Read the model definition and answer for the solid it produces. Units are mm, in the model's axes. Face numbers are marked on the shaded views. A direction names the side the tool comes from. Coordinates: 2 decimals unless noted, no trailing zeros. Write each loop counter-clockwise with the first axis right and the second up, starting at its lowest first coordinate (ties: lowest second). Pieces come first, ordered by that corner, then holes.
(1) Which of the six approach directions +Z, -Z, +X, -X, +Y, -Y give full straight-line access (tool end or side, diameter ignored) to the marked faces 5, 6, 7 and 8?
(2) Section A-A on y = 7.75 is taken. Write down the section's boundary in (x, z).
(3) Given pin 1 (0.5 mm diameter, centred on x = 5.5, y = 1, fed in from -Z); pin 2 (3 mm diameter, centred on y = 10, z = -1, fed in from +X); pin 3 (2 mm diameter, centred on x = 2, y = 8, fed in from -Z); pin 4 (6 mm diameter, centred on y = 1.5, z = 2, fed in from -X), each flat-ended and moving along its own axis, determine where each tip first touches the part or whether it passes through.
(4) Section B-B on z = 2.25 is taken. Write down the section's boundary in (x, y).
(5) The mould has two halves that part along X. Classify the marked faces 1, 2, 3 and 4: +X half, -X half, draft (parallel to the pull), parting line (faces both ways), or undercut.
(6) Section D-D on y = 5.25 is taken. Write down the section's boundary in (x, z), then the cut area to 3 significant figures.
(7) Section C-C on x = 7.25 is taken. Write down the section's boundary in (y, z).
(8) Find the intervals of material crossed by probe 1 along Y at (x, z) = (-2.55, -0.25); probe 2 along X at (y, z) = (3.25, -1.25); probe 3 along Z at (x, y) = (-1.5, 7.5), in increasing order.
Autodesk Inventor part; units mm, degrees
ref_plane "YZ Plane" through (0, 0, 0) normal (1, 0, 0) x (0, 1, 0)
ref_plane "XZ Plane" through (0, 0, 0) normal (0, 1, 0) x (-1, 0, 0)
ref_plane "XY Plane" through (0, 0, 0) normal (0, 0, 1) x (1, 0, 0)
sketch "Sketch1" plane through (0, 0, 0) normal (0, 1, 0) x (-1, 0, 0)
  circle A0 centre (6, 0) radius 1.6
  circle A1 centre (6, 0) radius 1.6
  circle A2 centre (-6, 0) radius 1.6
  circle A3 centre (-6, 0) radius 1.6
  line L0 (1, 2.75) -> (1, -2.75) construction
  line L1 (1, 2.75) -> (-1, 2.75)
  line L2 (-1, -2.75) -> (-1, 2.75) construction
  line L3 (-1, -2.75) -> (1, -2.75)
  line L4 (0, 2.75) -> (0, -2.75) construction
  line L5 (-1, -2.75) -> (-3, -2.75)
  line L6 (-3, -2.75) -> (-3, 2.75)
  line L7 (-3, 2.75) -> (-1, 2.75)
  line L8 (-1, 2.75) -> (-1, -2.75)
  line L9 (1, -2.75) -> (3, -2.75)
  line L10 (3, -2.75) -> (3, 2.75)
  line L11 (3, 2.75) -> (1, 2.75)
  line L12 (1, 2.75) -> (1, -2.75)
  line L13 (6, 0) -> (-6, 0) construction
  arc A4 (6, -2.5) -> (6, 2.5) centre (6, 0) ccw
  arc A5 (-6, 2.5) -> (-6, -2.5) centre (-6, 0) ccw
  line L14 (0, 2.75) -> (0, -2.75) construction
  arc A6 (4, 2.75) -> (-4, 2.75) centre (0, 2.75) ccw
  arc A7 (-4, -2.75) -> (4, -2.75) centre (0, -2.75) ccw
  line L15 (4, -2.75) -> (4, -2.5)
  line L16 (4, 2.5) -> (4, 2.75)
  line L17 (-4, 2.75) -> (-4, 2.5)
  line L18 (-4, -2.5) -> (-4, -2.75)
  line L19 (-6, -2.5) -> (-4, -2.5)
  line L20 (4, -2.5) -> (6, -2.5)
  line L21 (6, 2.5) -> (4, 2.5)
  line L22 (-4, 2.5) -> (-6, 2.5)
  point P0 (0, 0)
  point P1 (0, 0)
  point P2 (0, 0)
  point P3 (0, 0)
  point P4 (0, 0)
  point P5 (0, 0)
  dimension "d6" = 2
  dimension "d7" = 2
  dimension "d8" = 5
  dimension "d9" = 8
extrude "Extrusion1" add sketch "Sketch1" along normal blind 2 contours L11 L10 L9 L12 | L8 L5 L6 L7 | L20 L15 A7 L18 L19 A5 L22 L17 A6 L16 L21 A4
fillet "Fillet1" radius 1 4 edges at (4, 1, -2.5) (4, 1, 2.5) (-4, 1, -2.5) (-4, 1, 2.5)
sketch "Sketch3" plane through (0, 2, 0) normal (0, 1, 0) x (1, 0, 0)
  line L0 (1, -2.75) -> (-1, -2.75)
  line L1 (1, -2.75) -> (3, -2.75)
  line L2 (3, -2.75) -> (3, 2.75)
  line L3 (3, 2.75) -> (1, 2.75)
  line L4 (1, 2.75) -> (1, -2.75)
  line L5 (-1, -2.75) -> (-3, -2.75)
  line L6 (-3, -2.75) -> (-3, 2.75)
  line L7 (-3, 2.75) -> (-1, 2.75)
  line L8 (-1, 2.75) -> (-1, -2.75)
  point P0 (0, 0)
  dimension "d11" = 2
  dimension "d12" = 5.5
  dimension "d13" = 2
extrude "Extrusion2" add sketch "Sketch3" along normal blind 12
fillet "Fillet2" radius 0.5 6 edges at (2, 2, -2.75) (-2, 2, -2.75) (-3, 2, 0) (3, 2, 0) (2, 2, 2.75) (-2, 2, 2.75)
sketch "Sketch4" plane through (3, 14, 2.75) normal (1, 0, 0) x (0, 0, -1)
  line L0 (5.5, 0) -> (0.5, 0) construction
  line L1 (5.5, -12) -> (5.5, 0) construction
  line L2 (0.5, 0) -> (5.5, -12) construction
  line L3 (3, -6) -> (3, -9) construction
  line L4 (3, -6) -> (3.9934, -6) construction
  circle A0 centre (3, -9) radius 1.1
  circle A1 centre (3, -3) radius 1.1
  line L5 (0, 0) -> (5.5, 0)
  point P0 (2.75, -14)
  point P1 (52.5, -13.5)
  dimension "d17" = 3
  dimension "d18" = 2.2
extrude "Extrusion3" cut sketch "Sketch4" against normal blind 12
fillet "Fillet3" radius 1 4 edges at (2, 14, -2.75) (-2, 14, -2.75) (2, 14, 2.75) (-2, 14, 2.75)
properties part number "CarbonConnectorStabPCBConnector"
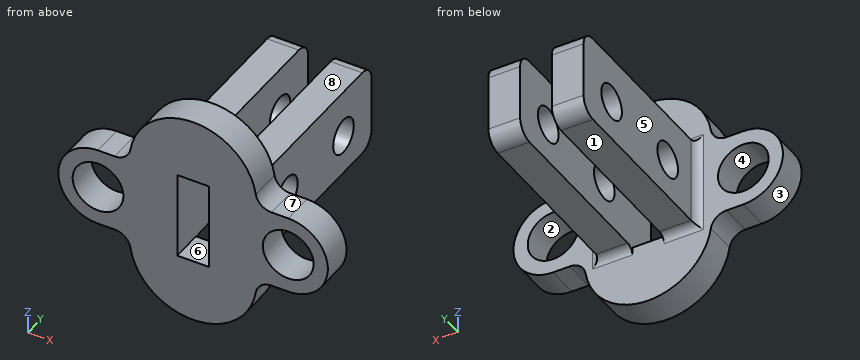
Response:
1. face 5: +Z, -Z, -X, +Y
1. face 6: +Y, -Y
1. face 7: +Z, +X, +Y, -Y
1. face 8: +Z, +X, -X, +Y
2. outline: (-3, -2.75) - (-1, -2.75) - (-1, 2.75) - (-3, 2.75) - close; (1, -2.75) - (3, -2.75) - (3, 2.75) - (1, 2.75) - close
3. pin 1: stops at z = -2.5
3. pin 2: stops at x = 3
3. pin 3: stops at z = -2.75
3. pin 4: stops at x = -8.5
4. outline: (-7.09, 0) - (-1, 0) - (-1, 13.87) - (-3, 13.87) - (-3, 2.5) arc R0.5 cw to (-3.5, 2) - (-7.09, 2) - close; (1, 0) - (7.09, 0) - (7.09, 2) - (3.5, 2) arc R0.5 cw to (3, 2.5) - (3, 13.87) - (1, 13.87) - close
5. face 1: draft
5. face 2: undercut
5. face 3: -X half
5. face 4: undercut
6. outline: (-3, -2.75) - (-1, -2.75) - (-1, -1.32) - (-3, -1.32) - close; (-3, 0.82) - (-1, 0.82) - (-1, 2.75) - (-3, 2.75) - close; (1, -2.75) - (3, -2.75) - (3, -1.32) - (1, -1.32) - close; (1, 0.82) - (3, 0.82) - (3, 2.75) - (1, 2.75) - close
6. area: 13.4 mm2
7. outline: (0, -2.17) - (2, -2.17) - (2, -1) - (0, -1) - close; (0, 1) - (2, 1) - (2, 2.17) - (0, 2.17) - close
8. probe 1: y = 0 to 3.9, 6.1 to 9.9, 12.1 to 14
8. probe 2: x = -3 to -1, 1 to 3
8. probe 3: z = -2.75 to 2.75
